Geometry: final body of the model. Coordinates: model frame, mm. A direction names the side the tool comes from. Round coordinates to 2 decimals unless told otherwise and drop trailing zeros. Answer in a Markdown table with one row per item. Add a question column.
from build123d import *

# Parameters (mm, degrees)
F0_W     = 32
F0_H     = 32
F1_DEPTH = 2.5
F2_W     = 29
F2_H     = 29
F4_W     = 27
F4_H     = 27
F6_R     = 1.5


with BuildPart() as f1:
    # F0 (on Top) → F1 (new body)
    with BuildSketch(Plane.XY):
        Rectangle(F0_W, F0_H)
    extrude(amount=F1_DEPTH)

    # F2 (on face) → F5 section 0
    with BuildSketch(Plane.XY.offset(2.5)):
        Rectangle(F2_W, F2_H)
    # F4 (on offset) → F5 section 1
    with BuildSketch(Plane.XY.offset(6)):
        Rectangle(F4_W, F4_H)
    loft()

    # F6
    f6_edges = [f1.edges().sort_by_distance(p)[0] for p in [
        (16, 16, 1.25),
        (16, -16, 1.25),
        (-16, 16, 1.25),
        (-16, -16, 1.25),
    ]]
    fillet(f6_edges, radius=F6_R)


solid = f1.part
1) Material intervals for line 1 along Z through (x, y) = (-15, -12); line 2 along Y through (x, z) = (-4.5, 4.5); line 3 along X through (y, z) = (-6, 4.25), sorted ascending. Write a range as from..to.
2) Contact query for a flat-ended pin moving along its axis: pin 1 Ø1 at (x, z) = (-12, 5.5) entering from -Y. Output: stop coordinate, or through.
3) Reachability of faces 1 (the flat face through (-1, -15, 2.5)), 2 (the flat face through (0, 0, 0)) from +Z, -Z, +X, -X, +Y, -Y: full face, straight path, thin tool, end or side. Return the list, or none.
Evaluation:
| question | item | result |
|---|---|---|
| 1 | line 1 | z = 0..2.5 |
| 1 | line 2 | y = -13.93..13.93 |
| 1 | line 3 | x = -14..14 |
| 2 | pin 1 | stops at y = -13.79 |
| 3 | face 1 | +Z |
| 3 | face 2 | -Z, +X, -X, +Y, -Y |
